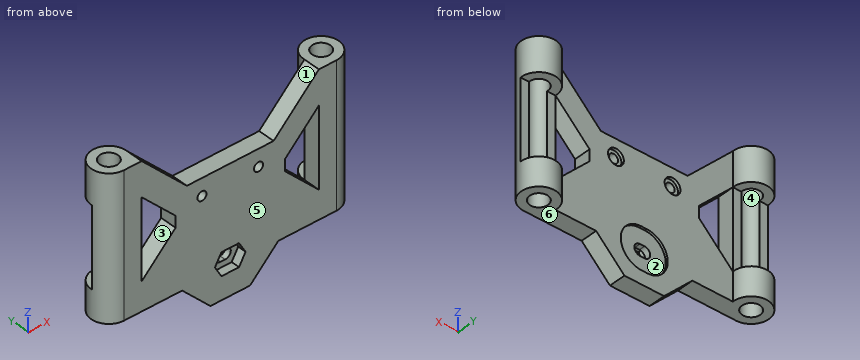
```python
from build123d import *

# Parameters (mm, degrees)
SKETCH_1_R             = 3.1
SKETCH_1_R_2           = 1.6
EXTRUDE_1_DEPTH        = 25
EXTRUDE_2_DEPTH        = 2.945
CUT_EXTRUDE_1_DEPTH    = 56.64644355
CUT_EXTRUDE_START      = -1.5
CUT_EXTRUDE_2844_DEPTH = 1.5
SKETCH_6_R             = 0.8
CUT_EXTRUDE_5_DEPTH    = 56.64644355
CUT_EXTRUDE_6_DEPTH    = 56.64644355
SKETCH_9_W             = 14
SKETCH_9_H             = 3.255
CUT_EXTRUDE_9_DEPTH    = 46.904396246
SKETCH_10_R            = 1.4
CUT_EXTRUDE_11_DEPTH   = 0.5
CUT_EXTRUDE_12_DEPTH   = 0.4


# Read off the part's stored shape, not the designer's step: 切除-螺母孔
with BuildPart() as part:
    # 草图1 → 凸台-拉伸1 (new body)
    # profile 1 of 3: a face of its own
    with BuildSketch(Plane.XY):
        with Locations((-46.507778168, 5.529205914)):
            Circle(SKETCH_1_R)
        with Locations((-46.507778168, 5.529205914)):
            Circle(SKETCH_1_R_2, mode=Mode.SUBTRACT)
    # profile 2 of 3: a face of its own
    with BuildSketch(Plane.XY):
        with BuildLine():
            ThreePointArc((-43.411655593, 5.374205914), (-44.371250611, 3.283042519), (-46.507778168, 2.429205914))
            Line((-46.507778168, 2.429205914), (-8.987778168, 2.429205914))
            ThreePointArc((-8.987778168, 2.429205914), (-11.124305724, 3.283042519), (-12.083900743, 5.374205914))
            Line((-12.083900743, 5.374205914), (-43.411655593, 5.374205914))
        make_face()
    # profile 3 of 3: a face of its own
    with BuildSketch(Plane.XY):
        with Locations((-8.987778168, 5.529205914)):
            Circle(SKETCH_1_R)
        with Locations((-8.987778168, 5.529205914)):
            Circle(SKETCH_1_R_2, mode=Mode.SUBTRACT)
    extrude(amount=EXTRUDE_1_DEPTH)

    # 草图2 → 凸台-拉伸2 (add)
    with BuildSketch(Plane(origin=(0, 5.374205914, 0), x_dir=(1, 0, 0), z_dir=(0, 1, 0))):
        Polygon((-19.247778168, 0), (-24.247778168, 5), (-31.247778168, 5), (-36.247778168, 0), align=None)
    extrude(amount=-EXTRUDE_2_DEPTH)

    # 草图3 → 切除-拉伸1 (cut, through all)
    with BuildSketch(Plane(origin=(0, 5.374205914, 0), x_dir=(1, 0, 0), z_dir=(0, 1, 0))):
        with BuildLine():
            Line((-28.147778168, 0), (-27.347778168, 0))
            ThreePointArc((-27.347778168, 0), (-26.347778168, -1), (-27.347778168, -2))
            Line((-27.347778168, -2), (-28.147778168, -2))
            ThreePointArc((-28.147778168, -2), (-29.147778168, -1), (-28.147778168, 0))
        make_face()
    extrude(amount=-CUT_EXTRUDE_1_DEPTH, mode=Mode.SUBTRACT)

    # Cut-Extrude 2844 outline → Cut-Extrude 2844 (cut)
    with BuildSketch(Plane(origin=(0, 2.429205914, 0), x_dir=(-1, 0, 0), z_dir=(0, -1, 0)).offset(CUT_EXTRUDE_START)):
        Polygon((25.038377091, -1), (26.193077629, -3), (29.302478706, -3), (30.457179245, -1), (29.302478706, 1), (26.193077629, 1), align=None)
        with BuildLine():
            Line((27.347778168, 0), (28.147778168, 0))
            ThreePointArc((28.147778168, 0), (29.147778168, -1), (28.147778168, -2))
            Line((28.147778168, -2), (27.347778168, -2))
            ThreePointArc((27.347778168, -2), (26.347778168, -1), (27.347778168, 0))
        make_face(mode=Mode.SUBTRACT)
    extrude(amount=CUT_EXTRUDE_2844_DEPTH, mode=Mode.SUBTRACT)

    # 草图6 → 切除-拉伸5 (cut, through all)
    with BuildSketch(Plane(origin=(0, 5.374205914, 0), x_dir=(1, 0, 0), z_dir=(0, 1, 0))):
        with Locations(Location((-32.747778168, -14, 0), (0, 0, 270))):
            Circle(SKETCH_6_R)
        with Locations(Location((-22.747778168, -14, 0), (0, 0, 270))):
            Circle(SKETCH_6_R)
    extrude(amount=-CUT_EXTRUDE_5_DEPTH, mode=Mode.SUBTRACT)

    # 草图7 → 切除-拉伸6 (cut, through all)
    with BuildSketch(Plane(origin=(0, 5.374205914, 0), x_dir=(1, 0, 0), z_dir=(0, 1, 0))):
        Polygon((-35.407778168, -17), (-43.407778168, -25), (-12.083900743, -25), (-20.083900743, -17), align=None)
        Polygon((-37.407778168, -13), (-37.407778168, -11), (-43.407778168, -5), (-43.407778168, -19), align=None)
        Polygon((-12.087778168, -5), (-18.087778168, -11), (-18.087778168, -13), (-12.087778168, -19), align=None)
    extrude(amount=-CUT_EXTRUDE_6_DEPTH, mode=Mode.SUBTRACT)

    # 草图9 → 切除-拉伸9 (cut, through all)
    with BuildSketch(Plane.ZY.offset(12.087778168)):
        with Locations((12, 7.001705914)):
            Rectangle(SKETCH_9_W, SKETCH_9_H)
    cut_extrude_9 = extrude(amount=-CUT_EXTRUDE_9_DEPTH, mode=Mode.SUBTRACT)

    # 镜向1: 切除-拉伸9 across plane
    add(cut_extrude_9.mirror(Plane(origin=(-27.747778168, 0, 0), x_dir=(0, 0, 1), z_dir=(1, 0, 0))), mode=Mode.SUBTRACT)

    # 草图10 → 切除-拉伸11 (cut)
    with BuildSketch(Plane(origin=(0, 5.374205914, 0), x_dir=(1, 0, 0), z_dir=(0, 1, 0))):
        with Locations(Location((-22.747778168, -14, 0), (0, 0, 270))):
            Circle(SKETCH_10_R)
        with Locations(Location((-32.747778168, -14, 0), (0, 0, 270))):
            Circle(SKETCH_10_R)
    extrude(amount=-CUT_EXTRUDE_11_DEPTH, mode=Mode.SUBTRACT)

    # 草图11 → 切除-拉伸12 (cut)
    with BuildSketch(Plane(origin=(0, 5.374205914, 0), x_dir=(1, 0, 0), z_dir=(0, 1, 0))):
        with BuildLine():
            Line((-27.247778168, -4.65), (-28.247778168, -4.65))
            ThreePointArc((-28.247778168, -4.65), (-31.897778168, -1), (-28.247778168, 2.65))
            Line((-28.247778168, 2.65), (-27.247778168, 2.65))
            ThreePointArc((-27.247778168, 2.65), (-23.597778168, -1), (-27.247778168, -4.65))
        make_face()
    extrude(amount=-CUT_EXTRUDE_12_DEPTH, mode=Mode.SUBTRACT)


solid = part.part
```
Here's how the part is built. I have some questions about the finished solid (model axes, mm). Face numbers are marked on the shaded views. A direction names the side the tool comes from. Coordinates: 2 decimals unless noted, no trailing zeros. Order: outer loops, then holes, each group sorted by start corner. A loop starts at its lowest first (then second) coordinate and runs counter-clockwise, first axis right, second up.
Item 1: If we section it at D-D, the plane y = 8: List the corners of the cut face in (x, z) for me.
Response values:
outline: (-48.38, 0) - (-44.64, 0) - (-44.64, 5) - (-48.38, 5) - close; (-48.38, 19) - (-44.64, 19) - (-44.64, 25) - (-48.38, 25) - close; (-10.86, 0) - (-7.12, 0) - (-7.12, 5) - (-10.86, 5) - close; (-10.86, 19) - (-7.12, 19) - (-7.12, 25) - (-10.86, 25) - close
Item 2: I need wall thicknesses on probe 1 along X at (y, z) = (3.3, 14); probe 2 along Z at (x, y) = (-45.5, 8); probe 3 along X at (y, z) = (2.9, 14). Which ranges of each line are inside material? Lowest first, please.
Response values:
probe 1: x = -48.66 to -43.41, -38.41 to -33.55, -31.95 to -23.55, -21.95 to -17.09, -12.09 to -6.83
probe 2: z = 0 to 5, 19 to 25
probe 3: x = -48.15 to -43.41, -38.41 to -33.55, -31.95 to -23.55, -21.95 to -17.09, -12.09 to -7.35
Item 3: Thinking about a two-plate mould opening in Y: for the marked faces 4, 5 and 6, which applies, pulls with the +Y half, pulls with the -Y half, needs draft (parallel to the pull), parting line crosses it, or undercut?
Response values:
face 4: undercut
face 5: pulls with the -Y half
face 6: needs draft
Item 4: If we section it at A-A, the plane z = 22: List the corners of the cut face in (x, y) for me.
Response values:
outline: (-46.51, 2.43) - (-40.41, 2.43) - (-40.41, 5.37) - (-43.41, 5.37) arc R3.1 ccw (long way) to start; (-15.08, 2.43) - (-8.99, 2.43) arc R3.1 ccw (long way) to (-12.08, 5.37) - (-15.08, 5.37) - close; hole circle Ø3.2 at (-46.51, 5.53); hole circle Ø3.2 at (-8.99, 5.53)
Item 5: Which directions (+Z, -Z, +X, -X, +Y, -Y) give clear straight access to the entire face, cutting with the end or side of a thin tool? Please do the marked faces 1, 2 and 3.
Response values:
face 1: +Z, +Y, -Y
face 2: +Y
face 3: +Y, -Y
Item 6: If we section it at C-C, the plane x = -15.5: List the corners of the cut face in (y, z) for me.
Response values:
outline: (2.43, 0) - (5.37, 0) - (5.37, 8.41) - (2.43, 8.41) - close; (2.43, 15.59) - (5.37, 15.59) - (5.37, 21.58) - (2.43, 21.58) - close
Item 7: If we section it at B-B, the plane z = 14: Give the number of separate pieces and of enclosed holes in the cut face, then the cut area to 3 significant figures.
Response values:
separate pieces: 5
enclosed holes: 0
area: 77.5 mm2
Item 8: I'm going to push flat-ended pins straight in: pin 1 Ø5 at (x, z) = (-22, 9.5) entering from +Y; pin 2 Ø0.6 at (x, y) = (-27.5, 4.5) entering from +Z; pin 3 Ø0.9 at (y, z) = (3.5, 10.5) entering from +X. Where does each tip first touch, or does it pass through?
Response values:
pin 1: stops at y = 5.37
pin 2: stops at z = 17
pin 3: stops at x = -6.32
